from build123d import *

# Parameters (mm, degrees)
SKETCH2_R           = 1.55
BOSS_EXTRUDE1_DEPTH = 3
FILLET1_R           = 2


with BuildPart() as part:
    # Sketch2 → Boss-Extrude1 (new body)
    with BuildSketch(Plane(origin=(0, 0, 0), x_dir=(1, 0, 0), z_dir=(0, 1, 0))):
        with BuildLine():
            Line((16.8134, 0), (16.8134, -70))
            Line((16.8134, -70), (26.8134, -70))
            Line((26.8134, -70), (26.8134, -40))
            Line((26.8134, -40), (31.5228, 0))
            ThreePointArc((31.5228, 0), (0, 31.5228), (-31.5228, 0))
            Line((-31.5228, 0), (-16.8134, 0))
            ThreePointArc((-16.8134, 0), (-14.522227787, 8.473211887), (-8.27315, 14.63712433))
            ThreePointArc((-8.27315, 14.63712433), (-5.923049404, 15.735561805), (-3.431948685, 16.459409096))
            ThreePointArc((-3.431948685, 16.459409096), (-3.966664912, 19.274974097), (-1.4, 18))
            ThreePointArc((-1.4, 18), (-1.583454565, 17.256092055), (-2.091748789, 16.682775745))
            ThreePointArc((-2.091748789, 16.682775745), (0, 16.8134), (2.091748789, 16.682775745))
            ThreePointArc((2.091748789, 16.682775745), (2.256092055, 19.416545435), (4.6, 18))
            ThreePointArc((4.6, 18), (4.274974097, 17.033335088), (3.431948685, 16.459409096))
            ThreePointArc((3.431948685, 16.459409096), (5.923049404, 15.735561805), (8.27315, 14.63712433))
            ThreePointArc((8.27315, 14.63712433), (14.522227787, 8.473211887), (16.8134, 0))
        make_face()
        with Locations((21.8134, -65.0887)):
            Circle(SKETCH2_R, mode=Mode.SUBTRACT)
        with Locations((21.8134, -58.3629)):
            Circle(SKETCH2_R, mode=Mode.SUBTRACT)
        with Locations((21.8134, -51.6371)):
            Circle(SKETCH2_R, mode=Mode.SUBTRACT)
        with Locations((21.8134, -44.9113)):
            Circle(SKETCH2_R, mode=Mode.SUBTRACT)
        with BuildLine():
            Line((-8.27315, 14.63712433), (8.27315, 14.63712433))
            ThreePointArc((8.27315, 14.63712433), (5.923049404, 15.735561805), (3.431948685, 16.459409096))
            ThreePointArc((3.431948685, 16.459409096), (2.73696162, 16.421769722), (2.091748789, 16.682775745))
            ThreePointArc((2.091748789, 16.682775745), (0, 16.8134), (-2.091748789, 16.682775745))
            ThreePointArc((-2.091748789, 16.682775745), (-2.73696162, 16.421769722), (-3.431948685, 16.459409096))
            ThreePointArc((-3.431948685, 16.459409096), (-5.923049404, 15.735561805), (-8.27315, 14.63712433))
        make_face()
        Polygon((31.5228, -70), (26.8134, -70), (26.8134, -40), (31.5228, 0), align=None)
    extrude(amount=BOSS_EXTRUDE1_DEPTH)

    # Fillet1
    fillet1_edges = [part.edges().sort_by_distance(p)[0] for p in [
        (-16.8134, 1.5, 0),
        (-31.5228, 1.5, 0),
        (31.5228, 1.5, 70),
        (16.8134, 1.5, 70),
        (8.27315, 1.5, -14.63712433),
        (-8.27315, 1.5, -14.63712433),
    ]]
    fillet(fillet1_edges, radius=FILLET1_R)


solid = part.part
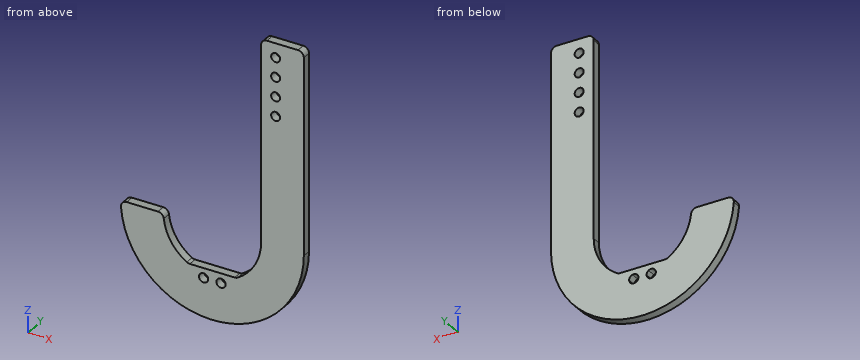
Input: part model. Units: mm. Frame: model coordinates. Coordinates: 2 decimals unless noted, no trailing zeros. Loops run counter-clockwise (first coordinate to the right, second up) from the corner with the lowest first, then second, coordinate; pieces in that order, holes last.
Q1. Cut plane A-A (y = 2.05). Output: boundary loops of the cut face in (x, z).
Q2. Material intervals for line 1 (X direction, y = 0.35, z = -17.5); line 2 (X direction, y = 2.15, z = -18); line 3 (X direction, y = 1.05, z = 2.5), sorted ascending.
Q3. Cut plane B-B (z = 31). Output: boundary loops of the cut face in (x, y), then the cut area to 3 significant figures.
Q4. Cut plane C-C (x = 0). Output: boundary loops of the cut face in (y, z), then the cut area to 3 significant figures.
Q5. Contact query for flat-ended pins moving along their axis: pin 1 (3.5 mm diameter, centred on x = -3, z = -18, fed in from -Y); pin 2 (1 mm diameter, centred on x = -19, y = 1.5, fed in from +Z). Output: stop coordinate, or through.
Working result:
1. outline: (-31.45, -2.14) arc R31.52 ccw to (31.52, 0) - (31.52, 68) arc R2 ccw to (29.52, 70) - (18.81, 70) arc R2 ccw to (16.81, 68) - (16.81, 0) arc R16.81 cw to (8.77, -14.34) arc R2 cw to (7.73, -14.64) - (-7.73, -14.64) arc R2 cw to (-8.77, -14.34) arc R16.81 cw to (-16.72, -1.79) arc R2 ccw to (-18.71, 0) - (-29.45, 0) arc R2 ccw to start; hole circle Ø3.2 at (-3, -18); hole circle Ø3.2 at (3, -18); hole circle Ø3.1 at (21.81, 44.91); hole circle Ø3.1 at (21.81, 51.64); hole circle Ø3.1 at (21.81, 58.36); hole circle Ø3.1 at (21.81, 65.09)
2. line 1: x = -26.22 to -4.52, -1.48 to 1.48, 4.52 to 26.22
2. line 2: x = -25.88 to -4.6, -1.4 to 1.4, 4.6 to 25.88
2. line 3: x = 16.81 to 31.52
3. outline: (16.81, 0) - (31.52, 0) - (31.52, 3) - (16.81, 3) - close
3. area: 44.1 mm2
4. outline: (0, -31.52) - (3, -31.52) - (3, -14.64) - (0, -14.64) - close
4. area: 50.7 mm2
5. pin 1: stops at y = 0
5. pin 2: stops at z = 0
